Geometry check sheet. Reference: the model listing, model coordinates, mm. A direction names the side the tool comes from. Give positions to 0.01 mm unless a question says otherwise; leave off trailing zeros. Loops run counter-clockwise (first coordinate to the right, second up) from the corner with the lowest first, then second, coordinate; pieces in that order, holes last.
1. Tool access check on faces 1 (the cylindrical face through (1.01, 28.86, -10.07)), 2 (the flat face through (1, 18, 3)), 3 (the flat face through (1, 30, -15)). Record the directions out of +Z, -Z, +X, -X, +Y, -Y that give a thin tool (end or side, any length) a straight path to the whole face; none if there is none.
2. Cross-section at A-A, the plane y = 0. Record the cut outline in (x, z), plus the area to 3 significant figures.
3. Material ranges on L1, parallel to Z at x = 1.5, y = 32.5; L2, parallel to Z at x = 1.6, y = 0; L3, parallel to Y at x = 0.9, z = 4, recorded low to high.
4. Cross-section at C-C, the plane y = 6.5. Record the cut outline in (x, z).
5. Cross-section at B-B, the plane x = 1. Record the cut outline in (y, z).
6. Cross-section at D-D, the plane y = -24. Record the cut outline in (x, z).
7. Release check for a two-part mould opening along Z. For faces 4 (the flat face through (1, 30, 15)), 5 (the cylindrical face through (0.99, 34.31, -14.4)), 6 (the cylindrical face through (1.01, 34.28, 3.57)) record: +Z half, -Z half, draft (parallel to the pull), parting line (faces both ways), or undercut.
8. Go/stop test with flat-tipped pins: pin 1 Ø0.6 at (x, y) = (0.5, 18.5) entering from +Z; pin 2 Ø0.6 at (x, y) = (1.5, 30.5) entering from -Z; pin 3 Ø0.6 at (x, y) = (1.5, 23.5) entering from -Z. Record where each tip stops, or that it passes through.
from build123d import *

# Parameters (mm, degrees)
SKETCH_1_R          = 30
EXTRUDE_1_DEPTH     = 2
SKETCH_2_R          = 5
CUT_EXTRUDE_1_DEPTH = 2
SKETCH_5_W          = 30
SKETCH_5_H          = 8.9
EXTRUDE_2_DEPTH     = 2
SKETCH_4_W          = 6
SKETCH_4_H          = 36.621783582
CUT_EXTRUDE_3_DEPTH = 2
FILLET_1_R          = 2
SKETCH_6_R          = 1.25
CUT_EXTRUDE_4_DEPTH = 2


with BuildPart() as part:
    # 草图1 → 凸台-拉伸1 (new body)
    with BuildSketch(Plane(origin=(0, 0, 0), x_dir=(0, 0, -1), z_dir=(1, 0, 0))):
        Circle(SKETCH_1_R)
    extrude(amount=EXTRUDE_1_DEPTH)

    # 草图2 → 切除-拉伸1 (cut)
    with BuildSketch(Plane(origin=(2, 0, 0), x_dir=(0, 0, -1), z_dir=(1, 0, 0))):
        Circle(SKETCH_2_R)
    extrude(amount=-CUT_EXTRUDE_1_DEPTH, mode=Mode.SUBTRACT)

    # 草图5 → 凸台-拉伸2 (add)
    with BuildSketch(Plane(origin=(2, 0, 0), x_dir=(0, 0, -1), z_dir=(1, 0, 0))):
        with Locations((0, 30.430762114)):
            Rectangle(SKETCH_5_W, SKETCH_5_H)
    extrude(amount=-EXTRUDE_2_DEPTH)

    # 草图4 → 切除-拉伸3 (cut)
    with BuildSketch(Plane(origin=(2, 0, 0), x_dir=(0, 0, -1), z_dir=(1, 0, 0))):
        with Locations((0, 20.061807767)):
            Rectangle(SKETCH_4_W, SKETCH_4_H)
    extrude(amount=-CUT_EXTRUDE_3_DEPTH, mode=Mode.SUBTRACT)

    # 圆角1
    fillet_1_edges = [part.edges().sort_by_distance(p)[0] for p in [
        (1, 25.980762114, 15),
        (1, 34.880762114, 15),
        (1, 34.880762114, -15),
        (1, 25.980762114, -15),
        (1, 34.880762114, -3),
        (1, 34.880762114, 3),
    ]]
    fillet(fillet_1_edges, radius=FILLET_1_R)

    # 草图6 → 切除-拉伸4 (cut)
    with BuildSketch(Plane(origin=(2, 0, 0), x_dir=(0, 0, -1), z_dir=(1, 0, 0))):
        with Locations((-10.455602866, 30.080762114)):
            Circle(SKETCH_6_R)
        with Locations((10.344397134, 30.080762114)):
            Circle(SKETCH_6_R)
    extrude(amount=-CUT_EXTRUDE_4_DEPTH, mode=Mode.SUBTRACT)


solid = part.part
Result:
1. face 1: +X, -X
1. face 2: +X, -X, +Y
1. face 3: -Z, +X, -X, +Y
2. outline: (0, -30) - (2, -30) - (2, -5) - (0, -5) - close; (0, 5) - (2, 5) - (2, 30) - (0, 30) - close
2. area: 100 mm2
3. L1: z = -15 to -3, 3 to 15
3. L2: z = -30 to -5, 5 to 30
3. L3: y = -29.73 to -3, 3 to 34.61
4. outline: (0, -29.29) - (2, -29.29) - (2, -3) - (0, -3) - close; (0, 3) - (2, 3) - (2, 29.29) - (0, 29.29) - close
5. outline: (4, -3) arc R5 cw (long way) to (4, 3) - (32.88, 3) arc R2 ccw to (34.88, 5) - (34.88, 13) arc R2 ccw to (32.88, 15) - (27.11, 15) arc R2 cw to (25.42, 15.94) arc R30 ccw (long way) to (25.42, -15.94) arc R2 cw to (27.11, -15) - (32.88, -15) arc R2 ccw to (34.88, -13) - (34.88, -5) arc R2 ccw to (32.88, -3) - close; hole circle Ø2.5 at (30.08, -10.34); hole circle Ø2.5 at (30.08, 10.46)
6. outline: (0, -18) - (2, -18) - (2, 18) - (0, 18) - close
7. face 4: +Z half
7. face 5: -Z half
7. face 6: undercut
8. pin 1: stops at z = 23.85
8. pin 2: stops at z = -15
8. pin 3: stops at z = -19.02
